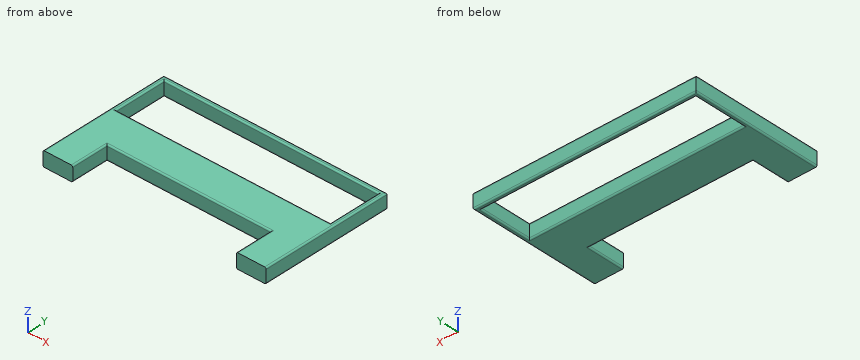
```python
from build123d import *

# Parameters (mm, degrees)
SKETCH1_W           = 1440
SKETCH1_H           = 350
BOSS_EXTRUDE1_DEPTH = 100
FILLET1_R           = 10


with BuildPart() as part:
    # Sketch1 → Boss-Extrude1 (new body)
    with BuildSketch(Plane.XY):
        Polygon((629.663880273, -500), (429.663880273, -500), (429.663880273, -250), (-670.336119727, -250), (-670.336119727, -500), (-870.336119727, -500), (-870.336119727, 380), (629.663880273, 380), align=None)
        with Locations((-120.336119727, 175)):
            Rectangle(SKETCH1_W, SKETCH1_H, mode=Mode.SUBTRACT)
    extrude(amount=BOSS_EXTRUDE1_DEPTH)

    # Fillet1
    fillet1_edges = [part.edges().sort_by_distance(p)[0] for p in [
        (429.663880273, -375, 0),
        (-120.336119727, -250, 0),
        (-670.336119727, -375, 0),
        (429.663880273, -375, 100),
        (629.663880273, -60, 100),
        (-840.336119727, 175, 0),
        (-120.336119727, 0, 0),
        (-120.336119727, 380, 100),
        (599.663880273, 175, 0),
        (-120.336119727, 350, 0),
        (-840.336119727, 175, 100),
        (-120.336119727, 0, 100),
        (599.663880273, 175, 100),
        (-120.336119727, 350, 100),
        (-870.336119727, -60, 100),
        (-670.336119727, -375, 100),
        (-120.336119727, -250, 100),
        (-870.336119727, -60, 0),
        (-120.336119727, 380, 0),
        (629.663880273, -60, 0),
    ]]
    fillet(fillet1_edges, radius=FILLET1_R)


solid = part.part
```
The listing builds one solid part. Answer for the finished solid, in the listing's coordinates (mm). Give positions to 0.01 mm unless a question says otherwise; leave off trailing zeros. Order: outer loops, then holes, each group sorted by start corner. A loop starts at its lowest first (then second) coordinate and runs counter-clockwise, first axis right, second up. Notation, with made-up numbers: (68, 82.25) - (98, 82.25) arc R22 cw to (98, 103.25) - close; hole circle Ø3 at (1.25, -13). An arc over 180 degrees is marked (long way). Use one line per item in the form item = value. Start each with the question number.
(1) A cutting plane is placed at D-D, the plane x = 470. Write down the section's boundary in (y, z), then the cut area to 3 significant figures.
(2) A cutting plane is placed at C-C, the plane z = 25.5. Write down the section's boundary in (x, y).
(3) A cutting plane is placed at A-A, the plane x = -486. Write down the section's boundary in (y, z), then the cut area to 3 significant figures.
(4) A cutting plane is placed at B-B, the plane y = 103. Write down the section's boundary in (x, z), then the cut area to 3 significant figures.
(5) Consider line 1 (X direction, y = -383.5, z = 15); line 2 (Y direction, x = -190.5, z = 69); line 3 (X direction, y = 238, z = 20.5). Determine where each line is inside the solid, lowest interval first. Write a range as from..to.
(6) A flat-ended cylindrical pin translates along its axis: pin 1 Ø12 at (x, z) = (-220.5, 16) entering from -Y. Find the tip coordinate at first contact, or state that the pin passes through.
Ans:
q1.outline = (-500, 0) - (-10, 0) arc R10 ccw to (0, 10) - (0, 90) arc R10 ccw to (-10, 100) - (-500, 100) - close; (350, 10) arc R10 ccw to (360, 0) - (370, 0) arc R10 ccw to (380, 10) - (380, 90) arc R10 ccw to (370, 100) - (360, 100) arc R10 ccw to (350, 90) - close
q1.area = 52,900 mm^2
q2.outline = (-870.34, -500) - (-670.34, -500) - (-670.34, -250) - (429.66, -250) - (429.66, -500) - (629.66, -500) - (629.66, 380) - (-870.34, 380) - close; hole (-840.34, 0) - (599.66, 0) - (599.66, 350) - (-840.34, 350) - close
q3.outline = (-250, 10) arc R10 ccw to (-240, 0) - (-10, 0) arc R10 ccw to (0, 10) - (0, 90) arc R10 ccw to (-10, 100) - (-240, 100) arc R10 ccw to (-250, 90) - close; (350, 10) arc R10 ccw to (360, 0) - (370, 0) arc R10 ccw to (380, 10) - (380, 90) arc R10 ccw to (370, 100) - (360, 100) arc R10 ccw to (350, 90) - close
q3.area = 27,800 mm^2
q4.outline = (-870.34, 10) arc R10 ccw to (-860.34, 0) - (-850.34, 0) arc R10 ccw to (-840.34, 10) - (-840.34, 90) arc R10 ccw to (-850.34, 100) - (-860.34, 100) arc R10 ccw to (-870.34, 90) - close; (599.66, 10) arc R10 ccw to (609.66, 0) - (619.66, 0) arc R10 ccw to (629.66, 10) - (629.66, 90) arc R10 ccw to (619.66, 100) - (609.66, 100) arc R10 ccw to (599.66, 90) - close
q4.area = 5,830 mm^2
q5.line_1 = -870.34..-670.34, 429.66..629.66
q5.line_2 = -250..0, 350..380
q5.line_3 = -870.34..-840.34, 599.66..629.66
q6.pin_1 = -250
